Design review of the part built by this model. Coordinates are the model's own, in mm. Give positions to 0.01 mm unless a question says otherwise; leave off trailing zeros. Loops run counter-clockwise (first coordinate to the right, second up) from the corner with the lowest first, then second, coordinate; pieces in that order, holes last. Notation, with made-up numbers: (18.25, 43) -> (50.25, 43) arc R20 cw to (50.25, 57) -> close; hole circle Ø9 at (35, 85.25). An arc over 180 degrees is marked (long way). Answer as CSV lines item,"result".
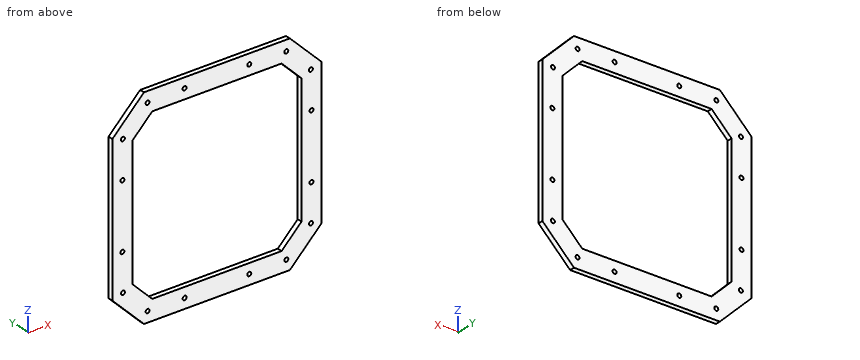
from build123d import *

# Parameters (mm, degrees)
SKETCH1_R           = 2
BOSS_EXTRUDE1_DEPTH = 5


with BuildPart() as part:
    # Sketch1 → Boss-Extrude1 (new body)
    with BuildSketch(Plane(origin=(0, 0, 0), x_dir=(1, 0, 0), z_dir=(0, 1, 0))):
        Polygon((105, -73.284271247), (105, 73.284271247), (73.284271247, 105), (-73.284271247, 105), (-105, 73.284271247), (-105, -73.284271247), (-73.284271247, -105), (73.284271247, -105), align=None)
        with Locations(Location((-95, 32.5, 0), (0, 0, 270))):
            Circle(SKETCH1_R, mode=Mode.SUBTRACT)
        with Locations(Location((-95, -32.5, 0), (0, 0, 90))):
            Circle(SKETCH1_R, mode=Mode.SUBTRACT)
        with Locations(Location((32.5, 95, 0), (0, 0, 270))):
            Circle(SKETCH1_R, mode=Mode.SUBTRACT)
        with Locations(Location((-32.5, 95, 0), (0, 0, 90))):
            Circle(SKETCH1_R, mode=Mode.SUBTRACT)
        with Locations(Location((-32.5, -95, 0), (0, 0, 270))):
            Circle(SKETCH1_R, mode=Mode.SUBTRACT)
        with Locations(Location((32.5, -95, 0), (0, 0, 90))):
            Circle(SKETCH1_R, mode=Mode.SUBTRACT)
        with Locations(Location((95, -32.5, 0), (0, 0, 270))):
            Circle(SKETCH1_R, mode=Mode.SUBTRACT)
        with Locations(Location((95, 32.5, 0), (0, 0, 90))):
            Circle(SKETCH1_R, mode=Mode.SUBTRACT)
        with Locations(Location((-94.445436483, -69.696699141, 0), (0, 0, 270))):
            Circle(SKETCH1_R, mode=Mode.SUBTRACT)
        with Locations(Location((-69.696699141, -94.445436483, 0), (0, 0, 90))):
            Circle(SKETCH1_R, mode=Mode.SUBTRACT)
        with Locations(Location((69.696699141, -94.445436483, 0), (0, 0, 270))):
            Circle(SKETCH1_R, mode=Mode.SUBTRACT)
        with Locations(Location((94.445436483, -69.696699141, 0), (0, 0, 90))):
            Circle(SKETCH1_R, mode=Mode.SUBTRACT)
        with Locations(Location((-94.445436483, 69.696699141, 0), (0, 0, 90))):
            Circle(SKETCH1_R, mode=Mode.SUBTRACT)
        with Locations(Location((-69.696699141, 94.445436483, 0), (0, 0, 270))):
            Circle(SKETCH1_R, mode=Mode.SUBTRACT)
        with Locations(Location((69.696699141, 94.445436483, 0), (0, 0, 90))):
            Circle(SKETCH1_R, mode=Mode.SUBTRACT)
        with Locations(Location((94.445436483, 69.696699141, 0), (0, 0, 270))):
            Circle(SKETCH1_R, mode=Mode.SUBTRACT)
        Polygon((65, 85), (85, 65), (85, -65), (65, -85), (-65, -85), (-85, -65), (-85, 65), (-65, 85), align=None, mode=Mode.SUBTRACT)
    extrude(amount=BOSS_EXTRUDE1_DEPTH)


solid = part.part
Q1. Clearance check with a flat-ended pin moving along its axis: pin 1 Ø3.5 at (x, z) = (-95, -32.5) entering from +Y. State where the tip first meets the part, or that it passes through.
Filled sheet:
pin 1,"passes through"
Q2. We need section C-C, the plane x = 80.5. State the section outline as (y, z) points, and give its area (3 significant figures).
Filled sheet:
outline,"(0, -97.78) -> (5, -97.78) -> (5, -69.5) -> (0, -69.5) -> close; (0, 69.5) -> (5, 69.5) -> (5, 97.78) -> (0, 97.78) -> close"
area,"283 mm^2"
Q3. We need section A-A, the plane z = 1. State the section outline as (x, y) points.
Filled sheet:
outline,"(-105, 0) -> (-85, 0) -> (-85, 5) -> (-105, 5) -> close; (85, 0) -> (105, 0) -> (105, 5) -> (85, 5) -> close"
Q4. We need section B-B, the plane y = 3.95. State how many separate pieces and enclosed holes the cut face has, and give its area (3 significant figures).
Filled sheet:
separate pieces,"1"
enclosed holes,"17"
area,"13,800 mm^2"
Q5. To check wall thickness, follow probe 1 along Z at (x, y) = (-64.5, 2.25); probe 2 along Z at (x, y) = (68.5, 0.6). State the ranges of each line that lie inside material, in increasing order. Write a range as from..to.
Filled sheet:
probe 1,"z = -105..-85, 85..105"
probe 2,"z = -105..-96.05, -92.84..-81.5, 81.5..92.84, 96.05..105"
